Input: part model. Units: mm. Frame: model coordinates. A direction names the side the tool comes from. Give positions to 0.01 mm unless a question says otherwise; leave off trailing zeros. Order: outer loops, then holes, each group sorted by start corner. A loop starts at its lowest first (then second) coordinate and runs counter-clockwise, first axis right, second up. Notation, with made-up numbers: (85, 87.25) - (138, 87.25) arc R19 ccw to (138, 97.25) - close; hole circle Ø10 at (-34.75, -34). An arc over 180 degrees is marked (long way). Answer in a Markdown table with one row per item. Add a question column.
1. Section query A-A on y = 57.15. Return loops of the section in (x, z), and give its area (3 significant figures).
2. Mould query, pull axis X, two halves, no side actions, for faces 1 (the face through (71, 83, 0)), 2 (the face through (0, 39, 3)), 3 (the face through (129.375, 20.302, 3.131)), 4 (the face through (152.4, 38, 3)). Classes: released by +X, released by -X, zero draft, split by the parting line, or undercut.
3. Section query B-B on x = 57.15. Return loops of the section in (y, z).
4. Section query C-C on x = 74.5. Return loops of the section in (y, z).
5. Access query for faces 5 (the face through (23, 76.2, 3)), 6 (the face through (93.33, 53.45, 3.13)). Directions: +Z, -Z, +X, -X, +Y, -Y. A direction counts if a zero-diameter tool reaches every point of the face in a straight line with its end or side. Return the directions, or none.
6. Ray query, line 1 (Y direction, x = 56, z = 3); line 2 (Y direction, x = 133.35, z = 2.75); line 3 (Y direction, x = 93.5, z = 4). Return the intervals inside material, ascending. Write a range as [from, to].
7. Contact query for flat-ended pins moving along their axis: pin 1 (9.5 mm diameter, centred on x = 133.35, y = 19.05, fed in from -Z); pin 2 (1 mm diameter, centred on x = 93.5, z = 4.5, fed in from +Y); pin 3 (6.5 mm diameter, centred on x = 19.05, y = 19.05, fed in from -Z); pin 4 (3 mm diameter, centred on y = 184, z = 2.5, fed in from +X). Output: stop coordinate, or through.
8. Section query D-D on z = 5. Count the separate pieces of the cut face and the enclosed holes in it, and give its area (3 significant figures).
```python
from build123d import *

# Parameters (mm, degrees)
BOSS_EXTRUDE1_DEPTH              = 6.35
F_21_64_0_32813_DIAMETER_HOLE1_D = 8.334502
LPATTERN1_COUNT                  = 4
LPATTERN1_PITCH                  = 38.1
LPATTERN1_COUNT_DIR2             = 2
LPATTERN1_PITCH_DIR2             = 38.1
F_21_64_0_32813_DIAMETER_HOLE2_D = 8.334502
LPATTERN2_COUNT                  = 3
LPATTERN2_PITCH                  = 38.1
LPATTERN2_COUNT_DIR2             = 2
LPATTERN2_PITCH_DIR2             = 38.1
FILLET1_R                        = 6.35


with BuildPart() as part:
    # Sketch2 → Boss-Extrude1 (new body)
    with BuildSketch(Plane.XY):
        Polygon((0, 0), (152.4, 0), (152.4, 76.2), (53.755193212, 208.590377648), (-7.34805801, 163.062005284), (57.373305284, 76.2), (0, 76.2), align=None)
    extrude(amount=BOSS_EXTRUDE1_DEPTH)

    # 21/64 (0.32813) Diameter Hole1 (through all)
    with Locations(Plane.XY.offset(6.35)):
        with Locations((133.35, 19.05)):
            f_21_64_0_32813_diameter_hole1 = Hole(F_21_64_0_32813_DIAMETER_HOLE1_D / 2)

    # LPattern1: 21_64 _0.32813_ Diameter Hole1 4 × 2
    with Locations(*[(-i * LPATTERN1_PITCH, j * LPATTERN1_PITCH_DIR2, 0) for i in range(LPATTERN1_COUNT) for j in range(LPATTERN1_COUNT_DIR2) if (i, j) != (0, 0)]):
        add(f_21_64_0_32813_diameter_hole1, mode=Mode.SUBTRACT)

    # 21/64 (0.32813) Diameter Hole2 (through all)
    with Locations(Plane.XY.offset(6.35)):
        with Locations((49.861473497, 181.932471751)):
            f_21_64_0_32813_diameter_hole2 = Hole(F_21_64_0_32813_DIAMETER_HOLE2_D / 2)

    # LPattern2: 21_64 _0.32813_ Diameter Hole2 3 × 2
    with Locations(*[Vector(0.5974852016253348, -0.8018799372965589, 0) * (i * LPATTERN2_PITCH) + Vector(-0.8018799372965586, -0.5974852016253351, 0) * (j * LPATTERN2_PITCH_DIR2) for i in range(LPATTERN2_COUNT) for j in range(LPATTERN2_COUNT_DIR2) if (i, j) != (0, 0)]):
        add(f_21_64_0_32813_diameter_hole2, mode=Mode.SUBTRACT)

    # Fillet1
    fillet1_edges = [part.edges().sort_by_distance(p)[0] for p in [
        (57.373305284, 76.2, 3.175),
    ]]
    fillet(fillet1_edges, radius=FILLET1_R)


solid = part.part
```
Answer:
| question | item | result |
|---|---|---|
| 1 | outline | (0, 0) - (14.88, 0) - (14.88, 6.35) - (0, 6.35) - close; (23.22, 0) - (52.98, 0) - (52.98, 6.35) - (23.22, 6.35) - close; (61.32, 0) - (91.08, 0) - (91.08, 6.35) - (61.32, 6.35) - close; (99.42, 0) - (129.18, 0) - (129.18, 6.35) - (99.42, 6.35) - close; (137.52, 0) - (152.4, 0) - (152.4, 6.35) - (137.52, 6.35) - close |
| 1 | area | 756 mm² |
| 2 | face 1 | zero draft |
| 2 | face 2 | released by -X |
| 2 | face 3 | undercut |
| 2 | face 4 | released by +X |
| 3 | outline | (0, 0) - (14.88, 0) - (14.88, 6.35) - (0, 6.35) - close; (23.22, 0) - (52.98, 0) - (52.98, 6.35) - (23.22, 6.35) - close; (61.32, 0) - (204.03, 0) - (204.03, 6.35) - (61.32, 6.35) - close |
| 4 | outline | (0, 0) - (147.66, 0) - (147.66, 6.35) - (0, 6.35) - close; (155.1, 0) - (180.75, 0) - (180.75, 6.35) - (155.1, 6.35) - close |
| 5 | face 5 | +Z, -Z, -X |
| 5 | face 6 | +Z, -Z |
| 6 | line 1 | y = [0, 15.04], [23.06, 53.14], [61.16, 205.58] |
| 6 | line 2 | y = [0, 14.88], [23.22, 52.98], [61.32, 101.77] |
| 6 | line 3 | y = [0, 15.27], [22.83, 53.37], [60.93, 117.12], [124.54, 155.25] |
| 7 | pin 1 | stops at z = 0 |
| 7 | pin 2 | stops at y = 155.92 |
| 7 | pin 3 | passes through |
| 7 | pin 4 | stops at x = 73.2 |
| 8 | separate pieces | 1 |
| 8 | enclosed holes | 14 |
| 8 | area | 21,300 mm² |
